from build123d import *

# Parameters (mm, degrees)
EXTRUDE_1_DEPTH = 2


with BuildPart() as part:
    # Model → 凸台-拉伸1 (new body)
    with BuildSketch(Plane.XY):
        Polygon((1417.579456282, 528.777626172), (1417.579456282, 523.704047707), (1419.079456282, 523.704047707), (1419.079456282, 513.704047707), (1417.579456282, 513.704047707), (1417.579456282, 514.474245762), (1412.579456282, 514.474245762), (1412.579456282, 509.474245762), (1417.579456282, 509.474245762), (1417.579456282, 478.155095762), (1419.079456282, 478.155095762), (1419.079456282, 468.155095762), (1417.579456282, 468.155095762), (1417.579456282, 467.474245762), (1412.579456282, 467.474245762), (1412.579456282, 462.474245762), (1407.579456282, 462.474245762), (1407.579456282, 461.474245762), (1397.579456282, 461.474245762), (1397.579456282, 462.474245762), (1392.579456282, 462.474245762), (1392.579456282, 461.474245762), (1382.579456282, 461.474245762), (1382.579456282, 462.474245762), (1377.579456282, 462.474245762), (1377.579456282, 467.474245762), (1372.579456282, 467.474245762), (1372.579456282, 468.155095762), (1371.079456282, 468.155095762), (1371.079456282, 478.155095762), (1372.579456282, 478.155095762), (1372.579456282, 509.474245762), (1377.579456282, 509.474245762), (1377.579456282, 514.474245762), (1372.579456282, 514.474245762), (1372.579456282, 513.704047707), (1371.079456282, 513.704047707), (1371.079456282, 523.704047707), (1372.579456282, 523.704047707), (1372.579456282, 528.777626172), align=None)
        with BuildLine():
            Line((1413.164476571, 491.917810861), (1413.164476571, 479.70647297))
            ThreePointArc((1413.164476571, 479.70647297), (1413.457369789, 478.999366189), (1414.164476571, 478.70647297))
            Line((1414.164476571, 478.70647297), (1414.555223152, 478.654447188))
            Line((1414.555223152, 478.654447188), (1414.555223152, 473.567457634))
            ThreePointArc((1414.555223152, 473.567457634), (1414.262329933, 472.860350852), (1413.555223152, 472.567457634))
            Line((1413.555223152, 472.567457634), (1410.947178647, 472.567457634))
            ThreePointArc((1410.947178647, 472.567457634), (1410.240071866, 472.274564415), (1409.947178647, 471.567457634))
            Line((1409.947178647, 471.567457634), (1409.947178647, 469.239749487))
            ThreePointArc((1409.947178647, 469.239749487), (1409.654285428, 468.532642706), (1408.947178647, 468.239749487))
            Line((1408.947178647, 468.239749487), (1382.420404996, 468.239749487))
            ThreePointArc((1382.420404996, 468.239749487), (1381.713298215, 468.532642706), (1381.420404996, 469.239749487))
            Line((1381.420404996, 469.239749487), (1381.420404996, 471.721090549))
            ThreePointArc((1381.420404996, 471.721090549), (1381.127511777, 472.428197331), (1380.420404996, 472.721090549))
            Line((1380.420404996, 472.721090549), (1376.569778947, 472.721090549))
            ThreePointArc((1376.569778947, 472.721090549), (1375.862672166, 473.013983768), (1375.569778947, 473.721090549))
            Line((1375.569778947, 473.721090549), (1375.569778947, 478.699498863))
            Line((1375.569778947, 478.699498863), (1376.305086446, 478.699498863))
            Line((1376.305086446, 478.699498863), (1376.305086446, 491.917810861))
            ThreePointArc((1376.305086446, 491.917810861), (1376.597979665, 492.624917642), (1377.305086446, 492.917810861))
            Line((1377.305086446, 492.917810861), (1412.164476571, 492.917810861))
            ThreePointArc((1412.164476571, 492.917810861), (1412.871583352, 492.624917642), (1413.164476571, 491.917810861))
        make_face(mode=Mode.SUBTRACT)
        Polygon((1382.679456282, 519.677225349), (1406.679456282, 519.677225349), (1406.679456282, 515.927225349), (1407.679456282, 515.927225349), (1407.679456282, 511.927225349), (1406.679456282, 511.927225349), (1406.679456282, 508.177225349), (1382.679456282, 508.177225349), align=None, mode=Mode.SUBTRACT)
        with BuildLine():
            Line((1411.462010719, 504.216917745), (1377.175235328, 504.216917745))
            ThreePointArc((1377.175235328, 504.216917745), (1376.468128547, 503.924024527), (1376.175235328, 503.216917745))
            Line((1376.175235328, 503.216917745), (1376.175235328, 497.276748548))
            ThreePointArc((1376.175235328, 497.276748548), (1376.468128547, 496.569641766), (1377.175235328, 496.276748548))
            Line((1377.175235328, 496.276748548), (1411.462010719, 496.276748548))
            ThreePointArc((1411.462010719, 496.276748548), (1412.1691175, 496.569641766), (1412.462010719, 497.276748548))
            Line((1412.462010719, 497.276748548), (1412.462010719, 503.216917745))
            ThreePointArc((1412.462010719, 503.216917745), (1412.1691175, 503.924024527), (1411.462010719, 504.216917745))
        make_face(mode=Mode.SUBTRACT)
    extrude(amount=EXTRUDE_1_DEPTH)


solid = part.part
Input: part model. Units: mm. Frame: model coordinates. A direction names the side the tool comes from. Coordinates: 2 decimals unless noted, no trailing zeros. Loops run counter-clockwise (first coordinate to the right, second up) from the corner with the lowest first, then second, coordinate; pieces in that order, holes last. Notation, with made-up numbers: (38, 58) -> (86, 58) arc R22 ccw to (86, 92) -> close; hole circle Ø6 at (-27.5, 62). An arc over 180 degrees is marked (long way). One line per item, written item: value.
(1) Pin query (flat end, axial travel): pin 1 Ø1 at (x, y) = (1406, 493.5) entering from -Z; pin 2 Ø1 at (y, z) = (486, 1.5) entering from -X. Return the tip coordinate at first contact, or that it passes through.
Answer below:
pin 1: stops at z = 0
pin 2: stops at x = 1372.58
(2) Draft query along X for faces 1 (the face through (1395, 508.177, 1)), 2 (the face through (1403, 461.474, 1)), 3 (the face through (1419.079, 519, 1)). Return one class per face: pulls with the +X half, pulls with the -X half, needs draft (parallel to the pull), parting line crosses it, or undercut.
Answer below:
face 1: undercut
face 2: needs draft
face 3: pulls with the +X half
(3) Cut plane A-A (y = 489.5). Output: boundary loops of the cut face in (x, z), then the cut area to 3 significant figures.
Answer below:
outline: (1372.58, 0) -> (1376.31, 0) -> (1376.31, 2) -> (1372.58, 2) -> close; (1413.16, 0) -> (1417.58, 0) -> (1417.58, 2) -> (1413.16, 2) -> close
area: 16.3 mm2
(4) Ray query, line 1 along Y through (x, z) = (1394.5, 1.2); line 2 along Y through (x, z) = (1387, 0.4); line 3 along X through (y, z) = (503, 1.35). Return the intervals inside material, ascending.
Answer below:
line 1: y = 462.47 to 468.24, 492.92 to 496.28, 504.22 to 508.18, 519.68 to 528.78
line 2: y = 461.47 to 468.24, 492.92 to 496.28, 504.22 to 508.18, 519.68 to 528.78
line 3: x = 1372.58 to 1376.18, 1412.46 to 1417.58
(5) Set-up query: faces 4 (the face through (1395, 519.677, 1)), 5 (the face through (1417.579, 494, 1)), 6 (the face through (1372, 478.155, 1)). Return all of +Z, -Z, +X, -X, +Y, -Y with unobstructed straight access to the full face (end or side cutting, diameter ignored); none if empty.
Answer below:
face 4: +Z, -Z
face 5: +Z, -Z, +X
face 6: +Z, -Z, -X
(6) Cut plane C-C (y = 513). Output: boundary loops of the cut face in (x, z).
Answer below:
outline: (1377.58, 0) -> (1382.68, 0) -> (1382.68, 2) -> (1377.58, 2) -> close; (1407.68, 0) -> (1412.58, 0) -> (1412.58, 2) -> (1407.68, 2) -> close
(7) Cut plane D-D (x = 1394). Output: boundary loops of the cut face in (y, z), then the cut area to 3 significant figures.
Answer below:
outline: (462.47, 0) -> (468.24, 0) -> (468.24, 2) -> (462.47, 2) -> close; (492.92, 0) -> (496.28, 0) -> (496.28, 2) -> (492.92, 2) -> close; (504.22, 0) -> (508.18, 0) -> (508.18, 2) -> (504.22, 2) -> close; (519.68, 0) -> (528.78, 0) -> (528.78, 2) -> (519.68, 2) -> close
area: 44.4 mm2
(8) Cut plane B-B (x = 1389). Output: boundary loops of the cut face in (y, z).
Answer below:
outline: (461.47, 0) -> (468.24, 0) -> (468.24, 2) -> (461.47, 2) -> close; (492.92, 0) -> (496.28, 0) -> (496.28, 2) -> (492.92, 2) -> close; (504.22, 0) -> (508.18, 0) -> (508.18, 2) -> (504.22, 2) -> close; (519.68, 0) -> (528.78, 0) -> (528.78, 2) -> (519.68, 2) -> close
